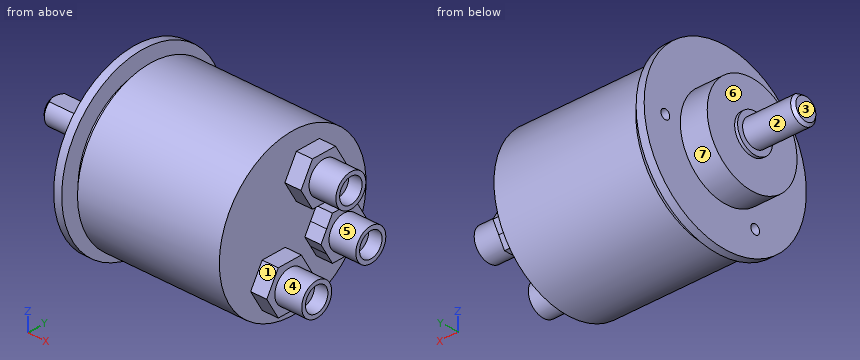
```python
from build123d import *

# Parameters (mm, degrees)
F0_R        = 5
F1_DEPTH    = 18.9
F2_W        = 21.1690347642
F2_H        = 4.931249544
F3_DEPTH    = 18.901
F4_T2_ANGLE = 359.64
F5_R        = 7
F6_DEPTH    = 1.1
F7_R        = 18
F8_DEPTH    = 10
F9_R        = 32.5
F10_DEPTH   = 3
F11_R       = 26
F12_DEPTH   = 3
F14_R       = 29.4
F15_DEPTH   = 52.8
F16_R       = 1.75
F17_DEPTH   = 3
F19_DEPTH   = 6
F20_R       = 6
F21_DEPTH   = 10
F22_R       = 4.5
F23_DEPTH   = 5


# Not quite as in the source:
# - a fillet or chamfer that OpenCascade refuses, or shapes differently, is made with other operations: its cross-section is extruded or revolved along the edge and cut away or added


with BuildPart() as f1:
    # F0 (on Right) → F1 (new body)
    with BuildSketch(Plane.YZ):
        Circle(F0_R)
    extrude(amount=-F1_DEPTH)

    # F2 (on Right) → F3 (cut, through all)
    with BuildSketch(Plane.YZ):
        with Locations((0.0764410943, 6.465624772)):
            Rectangle(F2_W, F2_H)
    extrude(amount=-F3_DEPTH, mode=Mode.SUBTRACT)

    # F4: chamfer of 1 on 1 edges, made by hand

    # F4_s1 → F4_t2 (revolve, cut)
    with BuildSketch(Plane(origin=(0, 0, 0), x_dir=(1, 0, 0), z_dir=(0, 0.9999950652, 0.0031415875))):
        with BuildLine():
            Line((-17.8717157288, -5.0282842712), (-18.9282842712, -3.9717157288))
            Line((-18.9282842712, -3.9717157288), (-18.9482842712, -3.9717157288))
            ThreePointArc((-18.9482842712, -3.9717157288), (-18.92, -4.4858578644), (-18.92, -5))
            Line((-18.92, -5), (-18.9, -5.02))
            ThreePointArc((-18.9, -5.02), (-18.3858578644, -5.02), (-17.8717157288, -5.0482842712))
            Line((-17.8717157288, -5.0482842712), (-17.8717157288, -5.0282842712))
        make_face()
    revolve(axis=Axis((-18.9, 0, 0), (1, 0, 0)), revolution_arc=F4_T2_ANGLE, mode=Mode.SUBTRACT)

    # F5 (on face) → F6 (join)
    with BuildSketch(Plane.YZ):
        Circle(F5_R)
    extrude(amount=F6_DEPTH)

    # F7 (on face) → F8 (join)
    with BuildSketch(Plane.YZ.offset(1.1)):
        Circle(F7_R)
    extrude(amount=F8_DEPTH)

    # F9 (on face) → F10 (join)
    with BuildSketch(Plane.YZ.offset(11.1)):
        Circle(F9_R)
    extrude(amount=F10_DEPTH)

    # F11 (on face) → F12 (join)
    with BuildSketch(Plane.YZ.offset(14.1)):
        Circle(F11_R)
    extrude(amount=F12_DEPTH)

    # F14 (on offset) → F15 (join, through all)
    with BuildSketch(Plane(origin=(69.9, 0, 0), x_dir=(0, -1, 0), z_dir=(-1, 0, 0))):
        Circle(F14_R)
    extrude(amount=F15_DEPTH)

    # F16 (on face) → F17 (cut)
    with BuildSketch(Plane(origin=(11.1, 0, 0), x_dir=(0, -1, 0), z_dir=(-1, 0, 0))):
        with Locations((-24, 0)):
            Circle(F16_R)
        with Locations((12, -20.7846096908)):
            Circle(F16_R)
        with Locations((12, 20.7846096908)):
            Circle(F16_R)
    extrude(amount=-F17_DEPTH, mode=Mode.SUBTRACT)

    # F18 (on face) → F19 (join)
    with BuildSketch(Plane.YZ.offset(69.9)):
        with BuildLine():
            ThreePointArc((21.0282031968, -10.574938038), (21.8274066017, -8.6454903731), (22.1, -6.57493798))
            ThreePointArc((22.1, -6.57493798), (21.8274066078, -4.5043856099), (21.0282032207, -2.5749379634))
            ThreePointArc((21.0282032207, -2.5749379634), (18.0999999917, 0.3532652551), (14.1, 1.42506202))
            ThreePointArc((14.1, 1.42506202), (10.1000001451, 0.3532653341), (7.1717969373, -2.5749376897))
            ThreePointArc((7.1717969373, -2.5749376897), (6.1, -6.5749379695), (7.1717969269, -10.5749382522))
            ThreePointArc((7.1717969269, -10.5749382522), (10.1000001361, -13.5031412888), (14.1, -14.57493798))
            ThreePointArc((14.1, -14.57493798), (18.099999971, -13.503141227), (21.0282031968, -10.574938038))
        make_face()
        with BuildLine():
            ThreePointArc((21.0282032207, -2.5749379634), (21.8274066078, -4.5043856099), (22.1, -6.57493798))
            ThreePointArc((22.1, -6.57493798), (21.8274066017, -8.6454903731), (21.0282031968, -10.574938038))
            Line((21.0282031968, -10.574938038), (23.337604307, -6.57493798))
            Line((23.337604307, -6.57493798), (21.0282032207, -2.5749379634))
        make_face()
        with BuildLine():
            ThreePointArc((14.1, 1.42506202), (18.0999999917, 0.3532652551), (21.0282032207, -2.5749379634))
            Line((21.0282032207, -2.5749379634), (18.7188021535, 1.42506202))
            Line((18.7188021535, 1.42506202), (14.1, 1.42506202))
        make_face()
        with BuildLine():
            Line((18.7188021535, -14.57493798), (21.0282031968, -10.574938038))
            ThreePointArc((21.0282031968, -10.574938038), (18.099999971, -13.503141227), (14.1, -14.57493798))
            Line((14.1, -14.57493798), (18.7188021535, -14.57493798))
        make_face()
        with BuildLine():
            ThreePointArc((7.1717969373, -2.5749376897), (10.1000001451, 0.3532653341), (14.1, 1.42506202))
            Line((14.1, 1.42506202), (9.4811978465, 1.42506202))
            Line((9.4811978465, 1.42506202), (7.1717969373, -2.5749376897))
        make_face()
        with BuildLine():
            Line((9.4811978465, -14.57493798), (14.1, -14.57493798))
            ThreePointArc((14.1, -14.57493798), (10.1000001361, -13.5031412888), (7.1717969269, -10.5749382522))
            Line((7.1717969269, -10.5749382522), (9.4811978465, -14.57493798))
        make_face()
        with BuildLine():
            ThreePointArc((7.1717969269, -10.5749382522), (6.1, -6.5749379695), (7.1717969373, -2.5749376897))
            Line((7.1717969373, -2.5749376897), (4.862395693, -6.57493798))
            Line((4.862395693, -6.57493798), (7.1717969269, -10.5749382522))
        make_face()
        Polygon((10.7188021535, 22.2), (1.4811978465, 22.2), (-3.137604307, 14.2), (1.4811978465, 6.2), (10.7188021535, 6.2), (15.337604307, 14.2), align=None)
        Polygon((-2.9811978465, -6.4), (-12.2188021535, -6.4), (-16.837604307, -14.4), (-12.2188021535, -22.4), (-2.9811978465, -22.4), (1.637604307, -14.4), align=None)
    extrude(amount=F19_DEPTH)

    # F20 (on face) → F21 (join)
    with BuildSketch(Plane.YZ.offset(75.9)):
        with Locations((6.1, 14.2)):
            Circle(F20_R)
        with Locations((14.1, -6.57493798)):
            Circle(F20_R)
        with Locations((-7.6, -14.4)):
            Circle(F20_R)
    extrude(amount=F21_DEPTH)

    # F22 (on face) → F23 (cut)
    with BuildSketch(Plane.YZ.offset(85.9)):
        with Locations((6.1, 14.2)):
            Circle(F22_R)
        with Locations((-7.6, -14.4)):
            Circle(F22_R)
        with Locations((14.1, -6.57493798)):
            Circle(F22_R)
    extrude(amount=-F23_DEPTH, mode=Mode.SUBTRACT)


solid = f1.part
```
Geometry check sheet. Reference: the model listing, model coordinates, mm. Face numbers are marked on the shaded views. A direction names the side the tool comes from. Round coordinates to 2 decimals unless told otherwise and drop trailing zeros. Loops run counter-clockwise (first coordinate to the right, second up) from the corner with the lowest first, then second, coordinate; pieces in that order, holes last. Notation, with made-up numbers: (47, -26.75) - (55, -26.75) arc R27 cw to (55, 6.25) - close; hole circle Ø5 at (-30, -38.5). An arc over 180 degrees is marked (long way). Write item = value, one per line. Start each with the question number.
1. Section check D-D on x = 4.5. Enter the section's corners in (y, z), then the cut area to 3 significant figures.
2. Mould release check, pull along Z, two halves, no side actions. Record for the marked faces 5, 6 and 7: released by +Z, released by -Z, zero draft, split by the parting line, or undercut.
3. Thickness scan on line 1 (X direction, y = -18.5, z = -20.5); line 2 (X direction, y = 23, z = -5); line 3 (X direction, y = -5, z = -4.5). Record the ranges inside material, lowest first.
4. Section check C-C on z = 16.5. Enter the section's corners in (x, y).
5. Set-up check for the marked faces 1, 2, 3 and 4: record each of +Z, -Z, +X, -X, +Y, -Y from which the full face is reachable in a straight line by a thin tool's end or side.
6. Section check A-A on y = 27.5. Enter the section's corners in (x, z), then the cut area to 3 significant figures.
7. Depth check by flat-ended pin: pin 1 (12 mm diameter, centred on x = 65, z = 23.5, fed in from +Y); pin 2 (2 mm diameter, centred on x = 67.5, y = 3.5, fed in from -Z); pin 3 (8 mm diameter, centred on x = 29.5, z = -22, fed in from -Y); pin 4 (19.5 mm diameter, centred on y = 9, z = 0.5, fed in from -X). Enter the tip coordinate at first touch or a pass-through.
8. Section check B-B on y = -24.5. Enter the section's corners in (x, z).
Working result:
q1.outline = circle Ø36 at (0, 0)
q1.area = 1,020 mm^2
q2.face_5 = undercut
q2.face_6 = zero draft
q2.face_7 = split by the parting line
q3.line_1 = 11.1 to 14.1, 17.1 to 69.9
q3.line_2 = 11.1 to 69.9
q3.line_3 = 0 to 69.9
q4.outline = (1.1, -7.19) - (11.1, -7.19) - (11.1, -28) - (14.1, -28) - (14.1, -20.09) - (17.1, -20.09) - (17.1, -24.33) - (69.9, -24.33) - (69.9, -1.81) - (75.9, -1.81) - (75.9, 0.56) - (85.9, 0.56) - (85.9, 2.23) - (80.9, 2.23) - (80.9, 9.97) - (85.9, 9.97) - (85.9, 11.64) - (75.9, 11.64) - (75.9, 14.01) - (69.9, 14.01) - (69.9, 24.33) - (17.1, 24.33) - (17.1, 20.09) - (14.1, 20.09) - (14.1, 28) - (11.1, 28) - (11.1, 7.19) - (1.1, 7.19) - close
q5.face_1 = +Z, +X, -Y
q5.face_2 = -X
q5.face_3 = +Z, -Z, -X, +Y, -Y
q5.face_4 = +X
q6.outline = (11.1, -17.32) - (14.1, -17.32) - (14.1, 17.32) - (11.1, 17.32) - close; (17.1, -10.4) - (69.9, -10.4) - (69.9, 10.4) - (17.1, 10.4) - close
q6.area = 1,200 mm^2
q7.pin_1 = 23.62
q7.pin_2 = -29.29
q7.pin_3 = -23.25
q7.pin_4 = -18.9
q8.outline = (11.1, -21.35) - (14.1, -21.35) - (14.1, -8.7) - (17.1, -8.7) - (17.1, -16.25) - (69.9, -16.25) - (69.9, 16.25) - (17.1, 16.25) - (17.1, 8.7) - (14.1, 8.7) - (14.1, 21.35) - (11.1, 21.35) - close
